Verification items for the finished model (mm, model axes). A direction names the side the tool comes from. Round coordinates to 2 decimals unless told otherwise and drop trailing zeros. Order: outer loops, then holes, each group sorted by start corner. A loop starts at its lowest first (then second) coordinate and runs counter-clockwise, first axis right, second up. Notation, with made-up numbers: M 88.25,1.5 L 129.25,1.5 A37 cw 129.25,38.5 Z; hole C 28.25,-20.75 d5. An arc over 180 degrees is marked long. One line per item, written item: value. Start each with the question number.
from build123d import *

# Parameters (mm, degrees)
SKETCH1_W                       = 100
SKETCH1_H                       = 100
BASE_FLANGE1_DEPTH              = 2.5
EDGE_FLANGE1_STRIP_W            = 16
EDGE_FLANGE1_STRIP_H            = 2.5
EDGE_FLANGE1_STRIP_CUT_DEPTH    = 83
EDGE_FLANGE1_RELIEF_W           = 17.25
EDGE_FLANGE1_RELIEF_H           = 1.25
EDGE_FLANGE1_RELIEF_CUT_DEPTH   = 2.5
EDGE_FLANGE1_DEPTH              = 83
EDGE_FLANGE2_STRIP_W            = 16
EDGE_FLANGE2_STRIP_H            = 2.5
EDGE_FLANGE2_STRIP_CUT_DEPTH    = 100
EDGE_FLANGE2_DEPTH              = 100
EDGE_FLANGE3_STRIP_W            = 16
EDGE_FLANGE3_STRIP_H            = 2.5
EDGE_FLANGE3_STRIP_CUT_DEPTH    = 50
EDGE_FLANGE3_RELIEF_W           = 17.25
EDGE_FLANGE3_RELIEF_H           = 1.25
EDGE_FLANGE3_RELIEF_CUT_DEPTH   = 2.5
EDGE_FLANGE3_DEPTH              = 50
SKETCH17_W                      = 50
SKETCH17_H                      = 8.5
CUT_EXTRUDE1_DEPTH              = 8.5
CUT_EXTRUDE2_REACH              = 150.345
F_10_0MM_DOWEL_HOLE1_AT_2_COUNT = 2
F_10_0MM_DOWEL_HOLE1_AT_2_PITCH = 60
F_10_0MM_DOWEL_HOLE2_AT_2_COUNT = 2
F_10_0MM_DOWEL_HOLE2_AT_2_PITCH = 60
FILLET3_R                       = 3
FILLET4_R                       = 10


# Sheet-metal steps are written as plain solids
with BuildPart() as part:
    # Sketch1 → Base-Flange1 (new body)
    with BuildSketch(Plane.XY):
        Rectangle(SKETCH1_W, SKETCH1_H)
    extrude(amount=-BASE_FLANGE1_DEPTH)

    # Edge-Flange1 strip (across the edge) → Edge-Flange1 strip cut (cut)
    with BuildSketch(Plane(origin=(-41.5, -50, 0), x_dir=(0, 1, 0), z_dir=(1, 0, 0))):
        with Locations((-2.5, -1.25)):
            Rectangle(EDGE_FLANGE1_STRIP_W, EDGE_FLANGE1_STRIP_H)
    extrude(amount=EDGE_FLANGE1_STRIP_CUT_DEPTH, mode=Mode.SUBTRACT)

    # Edge-Flange1 relief (on the sheet) → Edge-Flange1 relief cut (cut)
    with BuildSketch(Plane(origin=(-41.5, -44.5, 0), x_dir=(0, 1, 0), z_dir=(0, 0, 1))):
        with Locations((-7.375, 0.625)):
            Rectangle(EDGE_FLANGE1_RELIEF_W, EDGE_FLANGE1_RELIEF_H)
        with Locations((-7.375, -83.625)):
            Rectangle(EDGE_FLANGE1_RELIEF_W, EDGE_FLANGE1_RELIEF_H)
    extrude(amount=-EDGE_FLANGE1_RELIEF_CUT_DEPTH, mode=Mode.SUBTRACT)

    # Edge-Flange1 section (across the edge) → Edge-Flange1 (add)
    with BuildSketch(Plane(origin=(-41.5, -50, 0), x_dir=(0, 1, 0), z_dir=(1, 0, 0))):
        with BuildLine():
            Line((0, 3), (0, 40))
            Line((0, 40), (2.5, 40))
            Line((2.5, 40), (2.5, 3))
            ThreePointArc((2.5, 3), (3.378679656, 0.878679656), (5.5, 0))
            Line((5.5, 0), (5.5, -2.5))
            ThreePointArc((5.5, -2.5), (1.610912703, -0.889087297), (0, 3))
        make_face()
    extrude(amount=EDGE_FLANGE1_DEPTH)

    # Edge-Flange2 strip (across the edge) → Edge-Flange2 strip cut (cut)
    with BuildSketch(Plane(origin=(50, -50, 0), x_dir=(-1, 0, 0), z_dir=(0, 1, 0))):
        with Locations((-2.5, -1.25)):
            Rectangle(EDGE_FLANGE2_STRIP_W, EDGE_FLANGE2_STRIP_H)
    edge_flange2_strip_cut = extrude(amount=EDGE_FLANGE2_STRIP_CUT_DEPTH, mode=Mode.SUBTRACT)

    # Edge-Flange2 section (across the edge) → Edge-Flange2 (add)
    with BuildSketch(Plane(origin=(50, -50, 0), x_dir=(-1, 0, 0), z_dir=(0, 1, 0))):
        with BuildLine():
            Line((0, 3), (0, 97.5))
            Line((0, 97.5), (2.5, 97.5))
            Line((2.5, 97.5), (2.5, 3))
            ThreePointArc((2.5, 3), (3.378679656, 0.878679656), (5.5, 0))
            Line((5.5, 0), (5.5, -2.5))
            ThreePointArc((5.5, -2.5), (1.610912703, -0.889087297), (0, 3))
        make_face()
    edge_flange2 = extrude(amount=EDGE_FLANGE2_DEPTH)

    # Edge-Flange3 strip (across the edge) → Edge-Flange3 strip cut (cut)
    with BuildSketch(Plane(origin=(47.5, -50, 47.5), x_dir=(0, 1, 0), z_dir=(0, 0, 1))):
        with Locations((-2.5, -1.25)):
            Rectangle(EDGE_FLANGE3_STRIP_W, EDGE_FLANGE3_STRIP_H)
    edge_flange3_strip_cut = extrude(amount=EDGE_FLANGE3_STRIP_CUT_DEPTH, mode=Mode.SUBTRACT)

    # Edge-Flange3 relief (on the sheet) → Edge-Flange3 relief cut (cut)
    with BuildSketch(Plane(origin=(47.5, -44.5, 47.5), x_dir=(0, 1, 0), z_dir=(-1, 0, 0))):
        with Locations((-7.375, 0.625)):
            Rectangle(EDGE_FLANGE3_RELIEF_W, EDGE_FLANGE3_RELIEF_H)
    edge_flange3_relief_cut = extrude(amount=-EDGE_FLANGE3_RELIEF_CUT_DEPTH, mode=Mode.SUBTRACT)

    # Edge-Flange3 section (across the edge) → Edge-Flange3 (add)
    with BuildSketch(Plane(origin=(47.5, -50, 47.5), x_dir=(0, 1, 0), z_dir=(0, 0, 1))):
        with BuildLine():
            Line((0, 3), (0, 30))
            Line((0, 30), (2.5, 30))
            Line((2.5, 30), (2.5, 3))
            ThreePointArc((2.5, 3), (3.378679656, 0.878679656), (5.5, 0))
            Line((5.5, 0), (5.5, -2.5))
            ThreePointArc((5.5, -2.5), (1.610912703, -0.889087297), (0, 3))
        make_face()
    edge_flange3 = extrude(amount=EDGE_FLANGE3_DEPTH)

    # Sketch17 → Cut-Extrude1 (cut)
    with BuildSketch(Plane(origin=(50, 0, 0), x_dir=(0, 0, -1), z_dir=(1, 0, 0))):
        with Locations((-22.5, -45.75)):
            Rectangle(SKETCH17_W, SKETCH17_H)
    cut_extrude1 = extrude(amount=-CUT_EXTRUDE1_DEPTH, mode=Mode.SUBTRACT)

    # Sketch18 → Cut-Extrude2 (cut, up to next)
    with BuildSketch(Plane(origin=(50, 0, 0), x_dir=(0, 0, -1), z_dir=(1, 0, 0)), mode=Mode.PRIVATE) as cut_extrude2_sk1:
        Polygon((-97.5, 50), (-97.5, -35), (-12.5, 50), align=None)
    cut_extrude2_tool1 = extrude(cut_extrude2_sk1.sketch, amount=-CUT_EXTRUDE2_REACH, mode=Mode.PRIVATE) & part.part
    cut_extrude2 = cut_extrude2_tool1.solids().sort_by_distance((50, 21.666667, 69.166667))[0]
    add(cut_extrude2, mode=Mode.SUBTRACT)

    # Sketch20 → Ø10.0mm Dowel Hole1 (revolve, cut)
    with BuildSketch(Plane(origin=(30, 30, 0), x_dir=(0, -1, 0), z_dir=(1, 0, 0))):
        Polygon((0, 0), (0, 2.5), (5, 2.5), (5, 0.025), (5.025, 0), align=None)
    f_10_0mm_dowel_hole1 = revolve(axis=Axis((30, 30, 6.35), (0, 0, -1)), mode=Mode.SUBTRACT)

    # Ø10.0mm Dowel Hole1 at 2: Ø10.0mm Dowel Hole1 ×2
    with Locations(*[(0, -i * F_10_0MM_DOWEL_HOLE1_AT_2_PITCH, 0) for i in range(1, F_10_0MM_DOWEL_HOLE1_AT_2_COUNT)]):
        add(f_10_0mm_dowel_hole1, mode=Mode.SUBTRACT)

    # Sketch22 → Ø10.0mm Dowel Hole2 (revolve, cut)
    with BuildSketch(Plane(origin=(30, -47.5, 17.5), x_dir=(0, 0, 1), z_dir=(1, 0, 0))):
        Polygon((0, 0), (0, 2.5), (5, 2.5), (5, 0.025), (5.025, 0), align=None)
    f_10_0mm_dowel_hole2 = revolve(axis=Axis((30, -41.15, 17.5), (0, -1, 0)), mode=Mode.SUBTRACT)

    # Ø10.0mm Dowel Hole2 at 2: Ø10.0mm Dowel Hole2 ×2
    with Locations(*[(0, 0, i * F_10_0MM_DOWEL_HOLE2_AT_2_PITCH) for i in range(1, F_10_0MM_DOWEL_HOLE2_AT_2_COUNT)]):
        add(f_10_0mm_dowel_hole2, mode=Mode.SUBTRACT)

    # Mirror3: Edge-Flange2 strip cut, Edge-Flange2, Edge-Flange3 strip cut, Edge-Flange3 relief cut, Edge-Flange3, Cut-Extrude1, Cut-Extrude2, Ø10.0mm Dowel Hole1, Ø10.0mm Dowel Hole2 across plane
    add(edge_flange2_strip_cut.mirror(Plane(origin=(0, 0, 0), x_dir=(0, 0, 1), z_dir=(1, 0, 0))), mode=Mode.SUBTRACT)
    add(edge_flange2.mirror(Plane(origin=(0, 0, 0), x_dir=(0, 0, 1), z_dir=(1, 0, 0))))
    add(edge_flange3_strip_cut.mirror(Plane(origin=(0, 0, 0), x_dir=(0, 0, 1), z_dir=(1, 0, 0))), mode=Mode.SUBTRACT)
    add(edge_flange3_relief_cut.mirror(Plane(origin=(0, 0, 0), x_dir=(0, 0, 1), z_dir=(1, 0, 0))), mode=Mode.SUBTRACT)
    add(edge_flange3.mirror(Plane(origin=(0, 0, 0), x_dir=(0, 0, 1), z_dir=(1, 0, 0))))
    add(cut_extrude1.mirror(Plane(origin=(0, 0, 0), x_dir=(0, 0, 1), z_dir=(1, 0, 0))), mode=Mode.SUBTRACT)
    add(cut_extrude2.mirror(Plane(origin=(0, 0, 0), x_dir=(0, 0, 1), z_dir=(1, 0, 0))), mode=Mode.SUBTRACT)
    add(f_10_0mm_dowel_hole1.mirror(Plane(origin=(0, 0, 0), x_dir=(0, 0, 1), z_dir=(1, 0, 0))), mode=Mode.SUBTRACT)
    add(f_10_0mm_dowel_hole2.mirror(Plane(origin=(0, 0, 0), x_dir=(0, 0, 1), z_dir=(1, 0, 0))), mode=Mode.SUBTRACT)

    # Mirror3 copy 1 sketch → Mirror3 copy 1 (revolve, cut)
    with BuildSketch(Plane(origin=(-30, -30, 0), x_dir=(0, -1, 0), z_dir=(-1, 0, 0))):
        Polygon((0, 0), (0, -2.5), (5, -2.5), (5, -0.025), (5.025, 0), align=None)
    revolve(axis=Axis((-30, -30, 6.35), (0, 0, 1)), mode=Mode.SUBTRACT)

    # Mirror3 copy 2 sketch → Mirror3 copy 2 (revolve, cut)
    with BuildSketch(Plane(origin=(-30, -47.5, 77.5), x_dir=(0, 0, 1), z_dir=(-1, 0, 0))):
        Polygon((0, 0), (0, -2.5), (5, -2.5), (5, -0.025), (5.025, 0), align=None)
    revolve(axis=Axis((-30, -41.15, 77.5), (0, 1, 0)), mode=Mode.SUBTRACT)

    # Fillet3
    fillet3_edges = [part.edges().sort_by_distance(p)[0] for p in [
        (48.75, -41.5, 47.5),
        (41.5, -41.5, -1.25),
        (-48.75, -41.5, 47.5),
        (-41.5, -41.5, -1.25),
    ]]
    fillet(fillet3_edges, radius=FILLET3_R)

    # Fillet4
    fillet4_edges = [part.edges().sort_by_distance(p)[0] for p in [
        (17.5, -48.75, 47.5),
        (17.5, -48.75, 97.5),
        (48.75, 50, 12.5),
        (48.75, -35, 97.5),
        (-17.5, -48.75, 97.5),
        (-17.5, -48.75, 47.5),
        (-48.75, -35, 97.5),
        (-48.75, 50, 12.5),
        (-41.5, -48.75, 40),
        (41.5, -48.75, 40),
    ]]
    fillet(fillet4_edges, radius=FILLET4_R)


solid = part.part
1. Section check A-A (z = 26). Record the cut outline in (x, y), and give its area (4 significant figures).
2. Section check B-B (y = 30). Record the cut outline in (x, z) (3 decimals).
3. Draft check along X on faces 1 (the face through (-42.4, -42.36, -1.27)), 2 (the face through (-20.35, -48.73, 94.49)), 3 (the face through (-31, -47.5, 72)), 4 (the face through (50, -8, 39)). Enter one of: released by +X, released by -X, zero draft, split by the parting line, or undercut.
4. Depth check by flat-ended pin: pin 1 (8 mm diameter, centred on x = 30, y = 30, fed in from -Z); pin 2 (3 mm diameter, centred on x = 30.5, y = 3, fed in from +Z); pin 3 (8 mm diameter, centred on x = -36, z = 68, fed in from +Y); pin 4 (4.5 mm diameter, centred on y = -46.5, z = 6, fed in from +X). Enter the tip coordinate at first touch or a pass-through.
5. Section check C-C (z = 77.5). Record the cut outline in (x, y) (3 decimals).
6. Tool access check on faces 5 (the face through (38.49, -48.73, 37.15)), 6 (the face through (-1, 3, 0)), 7 (the face through (-38.65, -48.73, 36.99)), 8 (the face through (-20.51, -48.73, 50.35)). Record the directions out of +Z, -Z, +X, -X, +Y, -Y that give a thin tool (end or side, any length) a straight path to the whole face; none if there is none.
7. Scan lines: line 1 along X through (y, z) = (-49, 17); line 2 along X through (y, z) = (15, 23.5); line 3 along X through (y, z) = (30, -0.9). Record each from-to range of solid material in increasing order.
8. Section check D-D (x = -19). Record the cut outline in (y, z).
Geometry check:
1. outline: M -50,-41.5 L -47.5,-41.5 L -47.5,36.5 L -50,36.5 Z; M -41.5,-50 L 41.5,-50 L 41.5,-47.5 L -41.5,-47.5 Z; M 47.5,-41.5 L 50,-41.5 L 50,36.5 L 47.5,36.5 Z
1. area: 597.5 mm²
2. outline: M -50,3 A5.5 ccw -44.5,-2.5 L -35,-2.5 L -35,-0.025 L -35.025,0 L -44.5,0 A3 cw -47.5,3 L -47.5,32.5 L -50,32.5 Z; M -25,-2.5 L 25,-2.5 L 25,-0.025 L 24.975,0 L -24.975,0 L -25,-0.025 Z; M 35,-2.5 L 44.5,-2.5 A5.5 ccw 50,3 L 50,32.5 L 47.5,32.5 L 47.5,3 A3 cw 44.5,0 L 35.025,0 L 35,-0.025 Z
3. face 1: released by -X
3. face 2: undercut
3. face 3: undercut
3. face 4: released by +X
4. pin 1: passes through
4. pin 2: stops at z = 0
4. pin 3: stops at y = -47.5
4. pin 4: stops at x = 41.5
5. outline: M -50,-44.5 A5.5 ccw -44.5,-50 L -35,-50 L -35,-47.525 L -35.025,-47.5 L -44.5,-47.5 A3 cw -47.5,-44.5 L -47.5,-15 L -50,-15 Z; M -25,-50 L -17.5,-50 L -17.5,-47.5 L -24.975,-47.5 L -25,-47.525 Z; M 17.5,-50 L 25,-50 L 25,-47.525 L 24.975,-47.5 L 17.5,-47.5 Z; M 35,-50 L 44.5,-50 A5.5 ccw 50,-44.5 L 50,-15 L 47.5,-15 L 47.5,-44.5 A3 cw 44.5,-47.5 L 35.025,-47.5 L 35,-47.525 Z
6. face 5: +X, +Y, -Y
6. face 6: +Z, +Y
6. face 7: -X, +Y, -Y
6. face 8: +Y, -Y
7. line 1: x = -41.5 to -34.97, -25.03 to 25.03, 34.97 to 41.5
7. line 2: x = -50 to -47.5, 47.5 to 50
7. line 3: x = -48.38 to -35, -25 to 25, 35 to 48.38
8. outline: M -50,3 A5.5 ccw -44.5,-2.5 L 50,-2.5 L 50,0 L -44.5,0 A3 cw -47.5,3 L -47.5,40 L -50,40 Z; M -50,52.23 L -47.5,52.23 L -47.5,92.77 L -50,92.77 Z
